Autodesk Inventor part; units mm, degrees
ref_plane "YZ Plane" through (0, 0, 0) normal (1, 0, 0) x (0, 1, 0)
ref_plane "XY Plane" through (0, 0, 0) normal (0, 0, 1) x (1, 0, 0)
sketch "Sketch2" plane through (0, 0, 0) normal (0, 0, 1) x (1, 0, 0)
  line L0 (-15, 1) -> (-15, 0)
  line L1 (-15, 0) -> (15, 0)
  line L2 (15, 0) -> (15, 1)
  line L3 (15, 1) -> (-15, 1)
  line L4 (-15, 1) -> (15, 0) construction
  line L5 (-15, 0) -> (15, 1) construction
  line L6 (-13.1, 1) -> (-12.85, 1)
  line L7 (-12.85, 1) -> (-12.85, 0.7)
  line L8 (-12.85, 0.7) -> (-13.1, 0.7)
  line L9 (-13.1, 0.7) -> (-13.1, 1)
  line L10 (0, 0) -> (0, 1)
  line L11 (12.85, 1) -> (12.85, 0.7)
  line L12 (12.85, 0.7) -> (13.1, 0.7)
  line L13 (13.1, 0.7) -> (13.1, 1)
  line L14 (-21, 0) -> (21, 0)
  point P0 (0, 0.5)
  point P1 (0, 0.5)
  dimension "d1" = 1
  dimension "d2" = 30
  dimension "d3" = 0.25
  dimension "d4" = 0.3
  dimension "d5" = 25.7
revolve "Revolution1" add sketch "Sketch2" angle 360 about axis through (-10, 0, 0) along (1, 0, 0) contours L3 L9 L8 L7 L10 L1 L0 | L10 L3 L11 L12 L13 L2 L1
ref_plane "Work Plane1" through (0, 1, 0) normal (0, 1, 0) x (-1, 0, 0)
sketch "Sketch3" plane through (0, 1, 0) normal (0, 1, 0) x (-1, 0, 0)
  circle A0 centre (3.75, 0) radius 0.55
  line L0 (0, 0.9388) -> (0, -0.9388)
  circle A1 centre (-3.75, 0) radius 0.55
  point P0 (0, 0)
  point P1 (0, 0)
  dimension "d10" = 1.1
  dimension "d11" = 7.5
extrude "Extrusion1" cut sketch "Sketch3" against normal through all
chamfer "Chamfer1" distance 0.5 angle 45 2 edges at (-15, -1, 0) (15, -1, 0)
properties part number "axle"
Work out the finished part from the listing and answer in its coordinate system (mm). Coordinates: 2 decimals unless noted, no trailing zeros. Loops run counter-clockwise (first coordinate to the right, second up) from the corner with the lowest first, then second, coordinate; pieces in that order, holes last. Notation, with made-up numbers: M 36,37.25 L 86,37.25 A22 cw 86,70.25 Z; hole C 7.5,-35.75 d8. An arc over 180 degrees is marked long. Answer in a Markdown table with one row per item. Add a question column.
1. Find section C-C, the plane x = -3.75. Write down the section's boundary in (y, z), then the cut area to 3 significant figures.
2. Find section B-B, the plane y = 0. Write down the section's boundary in (x, z), then the cut area to 3 significant figures.
3. Find section A-A, the plane z = 0. State how many separate pieces and enclosed holes the cut face has, then the cut area to 3 significant figures.
4. Consider L1, parallel to X at y = -0.1, z = 0.05; L2, parallel to X at y = 0.65, z = -0.65; L3, parallel to Y at x = -7, z = -0.05. Determine where each line is inside the solid, lowest interval first.
5. Find section D-D, the plane x = -9.75. Write down the section's boundary in (y, z), then the cut area to 3 significant figures.
6. The mould has two halves that part along X. Classify faces 1 (the cylindrical face through (-3.345, 0.014, 0.372)), 2 (the cylindrical face through (0, 0, 1)), 3 (the flat face through (-15, 0, 0)): pulls with the +X half, pulls with the -X half, needs draft (parallel to the pull), parting line crosses it, or undercut.
7. A flat-ended cylindrical pin translates along its axis: P1, Ø1, axis at y = 0.5, z = 0.5, coming from the +X side. Find the tip coordinate at first contact, or state that the pin passes through.
Reported:
| question | item | result |
|---|---|---|
| 1 | outline | M -0.84,-0.55 A1 ccw 0.84,-0.55 Z; M -0.84,0.55 L 0.84,0.55 A1 ccw Z |
| 1 | area | 1.06 mm^2 |
| 2 | outline | M -15,-0.5 L -14.5,-1 L -13.1,-1 L -13.1,-0.7 L -12.85,-0.7 L -12.85,-1 L 12.85,-1 L 12.85,-0.7 L 13.1,-0.7 L 13.1,-1 L 14.5,-1 L 15,-0.5 L 15,0.5 L 14.5,1 L 13.1,1 L 13.1,0.7 L 12.85,0.7 L 12.85,1 L -12.85,1 L -12.85,0.7 L -13.1,0.7 L -13.1,1 L -14.5,1 L -15,0.5 Z; hole C -3.75,0 d1.1; hole C 3.75,0 d1.1 |
| 2 | area | 57.3 mm^2 |
| 3 | separate pieces | 3 |
| 3 | enclosed holes | 0 |
| 3 | area | 54.8 mm^2 |
| 4 | L1 | x = -15 to -4.3, -3.2 to 3.2, 4.3 to 15 |
| 4 | L2 | x = -14.58 to -13.1, -12.85 to 12.85, 13.1 to 14.58 |
| 4 | L3 | y = -1 to 1 |
| 5 | outline | C 0,0 d2 |
| 5 | area | 3.14 mm^2 |
| 6 | face 1 | undercut |
| 6 | face 2 | needs draft |
| 6 | face 3 | pulls with the -X half |
| 7 | P1 | stops at x = 15 |
